For this review, take the finished solid that the model builds, in its own axes (mm). Face numbers are marked on the shaded views. Round coordinates to 2 decimals unless told otherwise and drop trailing zeros. Write each loop counter-clockwise with the first axis right and the second up, starting at its lowest first coordinate (ties: lowest second). Pieces come first, ordered by that corner, then holes. Notation, with made-up numbers: (69, -38) -> (85, -38) arc R18 ccw to (85, -19) -> close; hole circle Ø5 at (80, 57.5). An arc over 180 degrees is marked (long way). Write item = value, one per line. Start each with the question number.
```python
from build123d import *

# Parameters (mm, degrees)
BOSS_EXTRUDE1_DEPTH      = 234.95
SKETCH3_W                = 1.5875
SKETCH3_H                = 12.7
BOSS_EXTRUDE3_DEPTH      = 234.95
LPATTERN1_COUNT          = 15
LPATTERN1_PITCH          = 38.1
MIRROR1_COPY_1_SKETCH_W  = 1.5875
MIRROR1_COPY_1_SKETCH_H  = 12.7
MIRROR1_COPY_1_DEPTH     = 234.95
MIRROR1_COPY_2_SKETCH_W  = 1.5875
MIRROR1_COPY_2_SKETCH_H  = 12.7
MIRROR1_COPY_2_DEPTH     = 234.95
MIRROR1_COPY_3_SKETCH_W  = 1.5875
MIRROR1_COPY_3_SKETCH_H  = 12.7
MIRROR1_COPY_3_DEPTH     = 234.95
MIRROR1_COPY_4_SKETCH_W  = 1.5875
MIRROR1_COPY_4_SKETCH_H  = 12.7
MIRROR1_COPY_4_DEPTH     = 234.95
MIRROR1_COPY_5_SKETCH_W  = 1.5875
MIRROR1_COPY_5_SKETCH_H  = 12.7
MIRROR1_COPY_5_DEPTH     = 234.95
MIRROR1_COPY_6_SKETCH_W  = 1.5875
MIRROR1_COPY_6_SKETCH_H  = 12.7
MIRROR1_COPY_6_DEPTH     = 234.95
MIRROR1_COPY_7_SKETCH_W  = 1.5875
MIRROR1_COPY_7_SKETCH_H  = 12.7
MIRROR1_COPY_7_DEPTH     = 234.95
MIRROR1_COPY_8_SKETCH_W  = 1.5875
MIRROR1_COPY_8_SKETCH_H  = 12.7
MIRROR1_COPY_8_DEPTH     = 234.95
MIRROR1_COPY_9_SKETCH_W  = 1.5875
MIRROR1_COPY_9_SKETCH_H  = 12.7
MIRROR1_COPY_9_DEPTH     = 234.95
MIRROR1_COPY_10_SKETCH_W = 1.5875
MIRROR1_COPY_10_SKETCH_H = 12.7
MIRROR1_COPY_10_DEPTH    = 234.95
MIRROR1_COPY_11_SKETCH_W = 1.5875
MIRROR1_COPY_11_SKETCH_H = 12.7
MIRROR1_COPY_11_DEPTH    = 234.95
MIRROR1_COPY_12_SKETCH_W = 1.5875
MIRROR1_COPY_12_SKETCH_H = 12.7
MIRROR1_COPY_12_DEPTH    = 234.95
MIRROR1_COPY_13_SKETCH_W = 1.5875
MIRROR1_COPY_13_SKETCH_H = 12.7
MIRROR1_COPY_13_DEPTH    = 234.95
MIRROR1_COPY_14_SKETCH_W = 1.5875
MIRROR1_COPY_14_SKETCH_H = 12.7
MIRROR1_COPY_14_DEPTH    = 234.95
BOSS_EXTRUDE4_DEPTH      = 234.95
MIRROR2_START            = 577.835817532
MIRROR2_OUTLINE_W        = 1.5875
MIRROR2_OUTLINE_H        = 234.95
MIRROR2_DEPTH            = 12.700003838


# Read off the part's stored shape, not the designer's step: Mirror2
with BuildPart() as part:
    # Sketch1 → Boss-Extrude1 (new body)
    with BuildSketch(Plane.XY):
        with BuildLine():
            Line((19.050003843, -3.175), (555.624996157, -3.175))
            ThreePointArc((555.624996157, -3.175), (577.849996157, 19.05), (555.624996157, 41.275))
            Line((555.624996157, 41.275), (19.049996157, 41.275))
            ThreePointArc((19.049996157, 41.275), (-3.175, 19.049996157), (19.050003843, -3.175))
        make_face()
        with BuildLine():
            Line((19.049996157, 0), (555.624996157, 0))
            ThreePointArc((555.624996157, 0), (574.674996157, 19.05), (555.624996157, 38.1))
            Line((555.624996157, 38.1), (19.050000909, 38.1))
            ThreePointArc((19.050000909, 38.1), (0, 19.050002376), (19.049996157, 0))
        make_face(mode=Mode.SUBTRACT)
    extrude(amount=BOSS_EXTRUDE1_DEPTH)

    # Sketch3 → Boss-Extrude3 (add)
    with BuildSketch(Plane.XY):
        with Locations((19.843746157, 47.625)):
            Rectangle(SKETCH3_W, SKETCH3_H)
    boss_extrude3 = extrude(amount=BOSS_EXTRUDE3_DEPTH)

    # LPattern1: Boss-Extrude3 ×15
    with Locations(*[(i * LPATTERN1_PITCH, 0, 0) for i in range(1, LPATTERN1_COUNT)]):
        add(boss_extrude3)

    # Mirror1: Boss-Extrude3 across plane
    add(boss_extrude3.mirror(Plane.ZX.offset(19.05)))

    # Mirror1 copy 1 sketch → Mirror1 copy 1 (add)
    with BuildSketch(Plane(origin=(38.1, 38.1, 0), x_dir=(1, 0, 0), z_dir=(0, 0, 1))):
        with Locations((19.843746157, -47.625)):
            Rectangle(MIRROR1_COPY_1_SKETCH_W, MIRROR1_COPY_1_SKETCH_H)
    extrude(amount=MIRROR1_COPY_1_DEPTH)

    # Mirror1 copy 2 sketch → Mirror1 copy 2 (add)
    with BuildSketch(Plane(origin=(76.2, 38.1, 0), x_dir=(1, 0, 0), z_dir=(0, 0, 1))):
        with Locations((19.843746157, -47.625)):
            Rectangle(MIRROR1_COPY_2_SKETCH_W, MIRROR1_COPY_2_SKETCH_H)
    extrude(amount=MIRROR1_COPY_2_DEPTH)

    # Mirror1 copy 3 sketch → Mirror1 copy 3 (add)
    with BuildSketch(Plane(origin=(114.3, 38.1, 0), x_dir=(1, 0, 0), z_dir=(0, 0, 1))):
        with Locations((19.843746157, -47.625)):
            Rectangle(MIRROR1_COPY_3_SKETCH_W, MIRROR1_COPY_3_SKETCH_H)
    extrude(amount=MIRROR1_COPY_3_DEPTH)

    # Mirror1 copy 4 sketch → Mirror1 copy 4 (add)
    with BuildSketch(Plane(origin=(152.4, 38.1, 0), x_dir=(1, 0, 0), z_dir=(0, 0, 1))):
        with Locations((19.843746157, -47.625)):
            Rectangle(MIRROR1_COPY_4_SKETCH_W, MIRROR1_COPY_4_SKETCH_H)
    extrude(amount=MIRROR1_COPY_4_DEPTH)

    # Mirror1 copy 5 sketch → Mirror1 copy 5 (add)
    with BuildSketch(Plane(origin=(190.5, 38.1, 0), x_dir=(1, 0, 0), z_dir=(0, 0, 1))):
        with Locations((19.843746157, -47.625)):
            Rectangle(MIRROR1_COPY_5_SKETCH_W, MIRROR1_COPY_5_SKETCH_H)
    extrude(amount=MIRROR1_COPY_5_DEPTH)

    # Mirror1 copy 6 sketch → Mirror1 copy 6 (add)
    with BuildSketch(Plane(origin=(228.6, 38.1, 0), x_dir=(1, 0, 0), z_dir=(0, 0, 1))):
        with Locations((19.843746157, -47.625)):
            Rectangle(MIRROR1_COPY_6_SKETCH_W, MIRROR1_COPY_6_SKETCH_H)
    extrude(amount=MIRROR1_COPY_6_DEPTH)

    # Mirror1 copy 7 sketch → Mirror1 copy 7 (add)
    with BuildSketch(Plane(origin=(266.7, 38.1, 0), x_dir=(1, 0, 0), z_dir=(0, 0, 1))):
        with Locations((19.843746157, -47.625)):
            Rectangle(MIRROR1_COPY_7_SKETCH_W, MIRROR1_COPY_7_SKETCH_H)
    extrude(amount=MIRROR1_COPY_7_DEPTH)

    # Mirror1 copy 8 sketch → Mirror1 copy 8 (add)
    with BuildSketch(Plane(origin=(304.8, 38.1, 0), x_dir=(1, 0, 0), z_dir=(0, 0, 1))):
        with Locations((19.843746157, -47.625)):
            Rectangle(MIRROR1_COPY_8_SKETCH_W, MIRROR1_COPY_8_SKETCH_H)
    extrude(amount=MIRROR1_COPY_8_DEPTH)

    # Mirror1 copy 9 sketch → Mirror1 copy 9 (add)
    with BuildSketch(Plane(origin=(342.9, 38.1, 0), x_dir=(1, 0, 0), z_dir=(0, 0, 1))):
        with Locations((19.843746157, -47.625)):
            Rectangle(MIRROR1_COPY_9_SKETCH_W, MIRROR1_COPY_9_SKETCH_H)
    extrude(amount=MIRROR1_COPY_9_DEPTH)

    # Mirror1 copy 10 sketch → Mirror1 copy 10 (add)
    with BuildSketch(Plane(origin=(381, 38.1, 0), x_dir=(1, 0, 0), z_dir=(0, 0, 1))):
        with Locations((19.843746157, -47.625)):
            Rectangle(MIRROR1_COPY_10_SKETCH_W, MIRROR1_COPY_10_SKETCH_H)
    extrude(amount=MIRROR1_COPY_10_DEPTH)

    # Mirror1 copy 11 sketch → Mirror1 copy 11 (add)
    with BuildSketch(Plane(origin=(419.1, 38.1, 0), x_dir=(1, 0, 0), z_dir=(0, 0, 1))):
        with Locations((19.843746157, -47.625)):
            Rectangle(MIRROR1_COPY_11_SKETCH_W, MIRROR1_COPY_11_SKETCH_H)
    extrude(amount=MIRROR1_COPY_11_DEPTH)

    # Mirror1 copy 12 sketch → Mirror1 copy 12 (add)
    with BuildSketch(Plane(origin=(457.2, 38.1, 0), x_dir=(1, 0, 0), z_dir=(0, 0, 1))):
        with Locations((19.843746157, -47.625)):
            Rectangle(MIRROR1_COPY_12_SKETCH_W, MIRROR1_COPY_12_SKETCH_H)
    extrude(amount=MIRROR1_COPY_12_DEPTH)

    # Mirror1 copy 13 sketch → Mirror1 copy 13 (add)
    with BuildSketch(Plane(origin=(495.3, 38.1, 0), x_dir=(1, 0, 0), z_dir=(0, 0, 1))):
        with Locations((19.843746157, -47.625)):
            Rectangle(MIRROR1_COPY_13_SKETCH_W, MIRROR1_COPY_13_SKETCH_H)
    extrude(amount=MIRROR1_COPY_13_DEPTH)

    # Mirror1 copy 14 sketch → Mirror1 copy 14 (add)
    with BuildSketch(Plane(origin=(533.4, 38.1, 0), x_dir=(1, 0, 0), z_dir=(0, 0, 1))):
        with Locations((19.843746157, -47.625)):
            Rectangle(MIRROR1_COPY_14_SKETCH_W, MIRROR1_COPY_14_SKETCH_H)
    extrude(amount=MIRROR1_COPY_14_DEPTH)

    # Sketch4 → Boss-Extrude4 (add)
    with BuildSketch(Plane.XY):
        with BuildLine():
            Line((-3.16082137, 19.84375), (-15.86082137, 19.84375))
            Line((-15.86082137, 19.84375), (-15.86082137, 18.25625))
            Line((-15.86082137, 18.25625), (-3.16082137, 18.25625))
            ThreePointArc((-3.16082137, 18.25625), (-3.175, 19.05), (-3.16082137, 19.84375))
        make_face()
    extrude(amount=BOSS_EXTRUDE4_DEPTH)

    # Mirror2 outline → Mirror2 (add)
    with BuildSketch(Plane.YZ.offset(MIRROR2_START)):
        with Locations((19.05, 117.475)):
            Rectangle(MIRROR2_OUTLINE_W, MIRROR2_OUTLINE_H)
    extrude(amount=MIRROR2_DEPTH)


solid = part.part
```
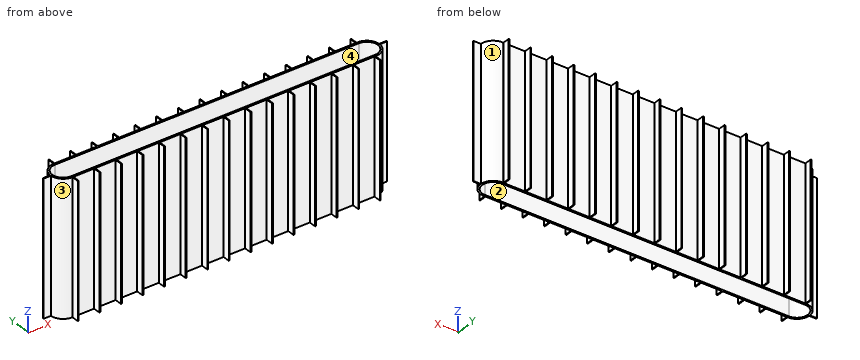
1. Wall thickness on L1, parallel to Y at x = 33.5, z = 141 (3 decimals); L2, parallel to X at y = 17, z = 209; L3, parallel to X at y = 18, z = 223: over which ranges is each line inside the solid? List them lowest first. Write a range as from..to.
2. Consider section A-A, the plane x = 380. Give the boundary of the cut face in (y, z) (3 decimals), then the cut area to 3 significant figures.
3. Consider section B-B, the plane y = 8. Give the boundary of the cut face in (x, z), then the cut area to 3 significant figures.
4. Clearance check with flat-ended pins moving along their axes: pin 1 Ø3 at (x, z) = (424.5, 172) entering from -Y (3 decimals); pin 2 Ø14 at (y, z) = (50.5, 158.5) entering from -X; pin 3 Ø14 at (y, z) = (-6.5, 170.5) entering from -X. State where each tip first meets the part, or that it passes through.
5. Draft analysis for pull direction X (two halves, no side actions). For the marked faces 1, 2, 3 and 4, state which applies: +X half, -X half, draft (parallel to the pull), parting line (faces both ways), or undercut.
Outcome:
q1.L1 = -3.175..0, 38.1..41.275
q1.L2 = -3.08..0.11, 574.56..577.76
q1.L3 = -3.15..0.03, 574.65..577.83
q2.outline = (-3.175, 0) -> (0, 0) -> (0, 234.95) -> (-3.175, 234.95) -> close; (38.1, 0) -> (41.275, 0) -> (41.275, 234.95) -> (38.1, 234.95) -> close
q2.area = 1,490 mm2
q3.outline = (-0.23, 0) -> (3.53, 0) -> (3.53, 234.95) -> (-0.23, 234.95) -> close; (571.14, 0) -> (574.91, 0) -> (574.91, 234.95) -> (571.14, 234.95) -> close
q3.area = 1,770 mm2
q4.pin_1 = -3.175
q4.pin_2 = 19.05
q4.pin_3 = 6.81
q5.face_1 = +X half
q5.face_2 = undercut
q5.face_3 = -X half
q5.face_4 = undercut
